Source: CAD feature listing. Evaluate the final solid. Frame: model axes, mm. A direction names the side the tool comes from. Give positions to 0.01 mm unless a question says otherwise; leave off trailing zeros. Loops run counter-clockwise (first coordinate to the right, second up) from the corner with the lowest first, then second, coordinate; pieces in that order, holes last.
from build123d import *

# Parameters (mm, degrees)
F0_R     = 41.275
F1_DEPTH = 3
F2_W     = 66
F2_H     = 20
F3_DEPTH = 3.001
F4_R     = 36.275
F4_W     = 66
F4_H     = 20
F5_DEPTH = 20


with BuildPart() as f1:
    # F0 (on Top) → F1 (new body)
    with BuildSketch(Plane.XY):
        Circle(F0_R)
    extrude(amount=F1_DEPTH)

    # F2 (on face) → F3 (cut, through all)
    with BuildSketch(Plane.XY.offset(3)):
        Rectangle(F2_W, F2_H)
    extrude(amount=-F3_DEPTH, mode=Mode.SUBTRACT)

    # F4 (on face) → F5 (join)
    with BuildSketch(Plane(origin=(0, 0, 0), x_dir=(1, 0, 0), z_dir=(0, 0, -1))):
        Circle(F4_R)
        with BuildLine():
            ThreePointArc((30.874747, -13), (0, -33.5), (-30.874747, -13))
            Line((-30.874747, -13), (30.874747, -13))
        make_face(mode=Mode.SUBTRACT)
        Rectangle(F4_W, F4_H, mode=Mode.SUBTRACT)
        with BuildLine():
            ThreePointArc((-30.874747, 13), (0, 33.5), (30.874747, 13))
            Line((30.874747, 13), (-30.874747, 13))
        make_face(mode=Mode.SUBTRACT)
    extrude(amount=F5_DEPTH)


solid = f1.part
1) Ray query, probe 1 along Y at (x, z) = (-22, -15.25); probe 2 along Y at (x, z) = (-27, -15.5); probe 3 along Z at (x, y) = (23.5, 19). Return the intervals inside material, ascending.
Checks:
probe 1: y = -28.84 to -25.26, -13 to -10, 10 to 13, 25.26 to 28.84
probe 2: y = -24.23 to -19.83, -13 to -10, 10 to 13, 19.83 to 24.23
probe 3: z = 0 to 3
2) Contact query for flat-ended pins moving along their axis: P1, Ø12, axis at y = -27, z = -13, coming from the -X side; P2, Ø10, axis at x = 14, y = 24.5, coming from the -Z side; P3, Ø1.5, axis at x = 24.5, z = -17, coming from the +Y side; P4, Ø1.5, axis at x = 30, y = -20.5, coming from the -Z side. Output: stop coordinate, or through.
Checks:
P1: stops at x = -29.58
P2: stops at z = 0
P3: stops at y = 27.42
P4: stops at z = -20
3) Cut plane B-B (x = 0). Return loops of the section in (y, z) (3 decimals), and give its area (3 significant figures).
Checks:
outline: (-41.275, 0) - (-36.275, 0) - (-36.275, -20) - (-33.5, -20) - (-33.5, 0) - (-13, 0) - (-13, -20) - (-10, -20) - (-10, 3) - (-41.275, 3) - close; (10, -20) - (13, -20) - (13, 0) - (33.5, 0) - (33.5, -20) - (36.275, -20) - (36.275, 0) - (41.275, 0) - (41.275, 3) - (10, 3) - close
area: 419 mm2
4) Reachability of faces 5 (the flat face through (-1, -18, 3)), 6 (the flat face through (0, 21, 0)), 7 (the flat face through (-33, 0, -8)) from +Z, -Z, +X, -X, +Y, -Y: full face, straight path, thin tool, end or side. Return the list, or none.
Checks:
face 5: +Z, +X, -X, +Y, -Y
face 6: -Z
face 7: +Z, -Z
5) Cut plane A-A (y = 0). Return loops of the section in (x, z) (3 decimals), and give its area (3 significant figures).
Checks:
outline: (-41.275, 0) - (-36.275, 0) - (-36.275, -20) - (-33, -20) - (-33, 3) - (-41.275, 3) - close; (33, -20) - (36.275, -20) - (36.275, 0) - (41.275, 0) - (41.275, 3) - (33, 3) - close
area: 181 mm2
6) Cut plane C-C (z = -9.25). Return loops of the section in (x, y) (3 decimals).
Checks:
outline: circle Ø72.55 at (0, 0); hole (-33, -10) - (33, -10) - (33, 10) - (-33, 10) - close; hole (-30.875, -13) arc R33.5 ccw to (30.875, -13) - close; hole (-30.875, 13) - (30.875, 13) arc R33.5 ccw to start
7) Cut plane D-D (x = 16). Return loops of the section in (y, z), and give its area (3 significant figures).
Checks:
outline: (-38.05, 0) - (-32.56, 0) - (-32.56, -20) - (-29.43, -20) - (-29.43, 0) - (-13, 0) - (-13, -20) - (-10, -20) - (-10, 3) - (-38.05, 3) - close; (10, -20) - (13, -20) - (13, 0) - (29.43, 0) - (29.43, -20) - (32.56, -20) - (32.56, 0) - (38.05, 0) - (38.05, 3) - (10, 3) - close
area: 413 mm2
8) Pull-direction query (Y, two-part tool) for faces 1 (the cylindrical face through (-8.948, -40.293, 1.479)), 2 (the flat face through (0, -21, 0)), 3 (the flat face through (33, 0, -8)), 4 (the flat face through (0, 11, -20)); classes: released by +Y, released by -Y, zero draft, split by the parting line, or undercut.
Checks:
face 1: split by the parting line
face 2: undercut
face 3: undercut
face 4: zero draft
